Answer from the drawing. Dimensions are ordinates in mm from the lowest x, y and z of the part. Round coordinates to 2 decimals unless told otherwise and drop trailing zeros. Loops run counter-clockwise (first coordinate to the right, second up) from the corner with the lowest first, then second, coordinate; pieces in that order, holes last.
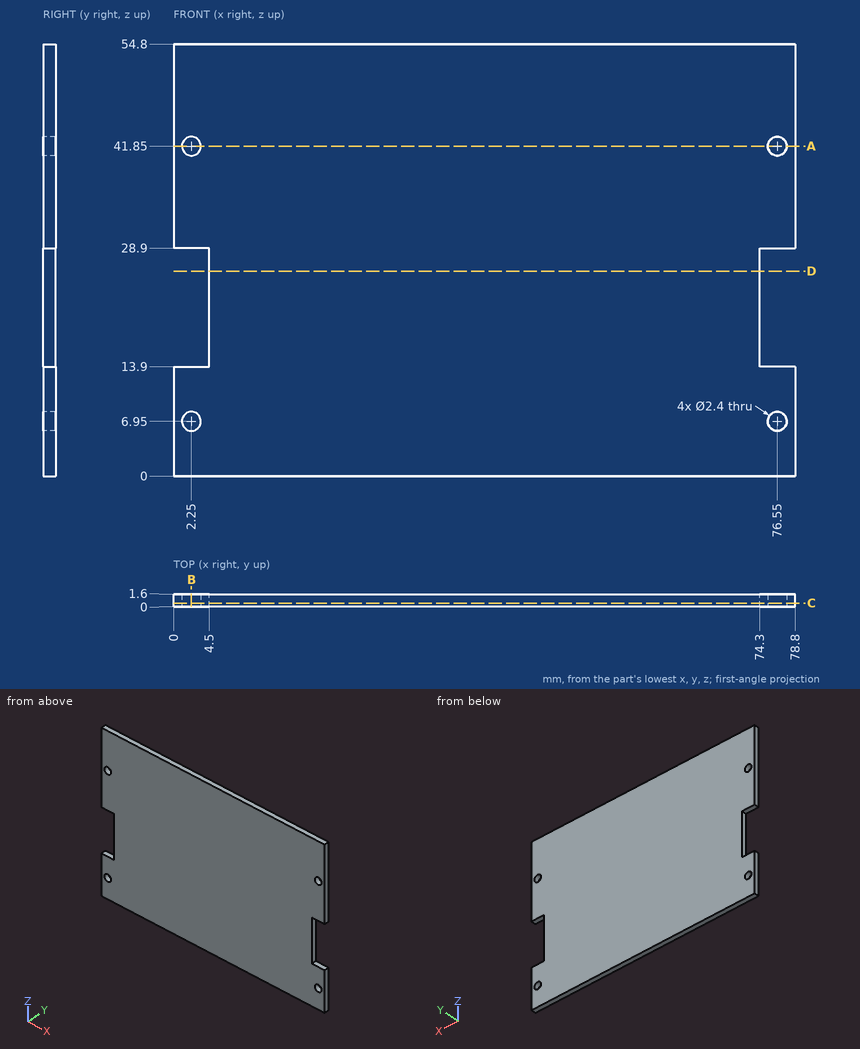
Item 1: Section C-C, the plane y = 0.45 is taken. Give the vertices of the cut face in (x, z), plus the area to 3 significant figures.
Item 2: Section D-D, the plane z = 26 is taken. Give the vertices of the cut face in (x, y).
Item 3: Straight lines are drawn through the part: line 1 (X direction, y = 0.5, z = 6.95); line 2 (Z direction, x = 2.25, y = 0.45); line 3 (X direction, y = 1.2, z = 26). For each, find the intervals that lie inside material, in ascending order.
Item 4: Section B-B, the plane x = 2.25 is taken. Give the vertices of the cut face in (y, z), plus the area to 3 significant figures.
Item 5: Section A-A, the plane z = 41.85 is taken. Give the vertices of the cut face in (x, y).
Item 6: This flat-tipped pin is pushed along its axis until it touches: P1, Ø0.8, axis at y = 1, z = 24, coming from the -X side. Where does it stop, or does it pass through?
Answer below:
1. outline: (0, 0) - (78.8, 0) - (78.8, 13.9) - (74.3, 13.9) - (74.3, 28.9) - (78.8, 28.9) - (78.8, 54.8) - (0, 54.8) - (0, 28.9) - (4.5, 28.9) - (4.5, 13.9) - (0, 13.9) - close; hole circle Ø2.4 at (2.25, 6.95); hole circle Ø2.4 at (2.25, 41.85); hole circle Ø2.4 at (76.55, 6.95); hole circle Ø2.4 at (76.55, 41.85)
1. area: 4,170 mm2
2. outline: (4.5, 0) - (74.3, 0) - (74.3, 1.6) - (4.5, 1.6) - close
3. line 1: x = 0 to 1.05, 3.45 to 75.35, 77.75 to 78.8
3. line 2: z = 0 to 5.75, 8.15 to 13.9, 28.9 to 40.65, 43.05 to 54.8
3. line 3: x = 4.5 to 74.3
4. outline: (0, 0) - (1.6, 0) - (1.6, 5.75) - (0, 5.75) - close; (0, 8.15) - (1.6, 8.15) - (1.6, 13.9) - (0, 13.9) - close; (0, 28.9) - (1.6, 28.9) - (1.6, 40.65) - (0, 40.65) - close; (0, 43.05) - (1.6, 43.05) - (1.6, 54.8) - (0, 54.8) - close
4. area: 56.0 mm2
5. outline: (0, 0) - (1.05, 0) - (1.05, 1.6) - (0, 1.6) - close; (3.45, 0) - (75.35, 0) - (75.35, 1.6) - (3.45, 1.6) - close; (77.75, 0) - (78.8, 0) - (78.8, 1.6) - (77.75, 1.6) - close
6. P1: stops at x = 4.5
